```python
from build123d import *

# Parameters (mm, degrees)
FILLET_1_R      = 2
CHAMFER_1_SIZE  = 0.5
CHAMFER_1_SIZE2 = 0.288675135
CHAMFER_2_SIZE  = 0.5
CHAMFER_2_SIZE2 = 0.288675135
SKETCH_2_R      = 17.5
SKETCH_2_R_2    = 10
EXTRUDE_1_DEPTH = 2
CHAMFER_3_SIZE  = 0.5
CHAMFER_4_SIZE  = 0.5
FILLET_2_R      = 0.25


with BuildPart() as part:
    # ｽｹｯﾁ1 → 回転1 (revolve)
    with BuildSketch(Plane(origin=(0, 0, 0), x_dir=(0, 0, -1), z_dir=(1, 0, 0)), mode=Mode.PRIVATE) as revolve_1_sk:
        Polygon((-9, 37.5), (-14, 32.5), (-14, 29), (-7, 29), (-7, 26), (-2, 26), (-2, 12), (3, 12), (3, 17.5), (0, 17.5), (0, 37.5), align=None)
    revolve(revolve_1_sk.sketch.rotate(Axis((0, 0, 26.899509804), (0, 0, -1)), 90), axis=Axis((0, 0, 26.899509804), (0, 0, -1)))

    # ﾌｨﾚｯﾄ1
    fillet_1_edges = [part.edges().sort_by_distance(p)[0] for p in [
        (-17.5, 0, 0),
        (-32.5, 0, 14),
    ]]
    fillet(fillet_1_edges, radius=FILLET_1_R)

    # 面取り1
    chamfer_1_edges = [part.edges().sort_by_distance(p)[0] for p in [
        (-29, 0, 14),
    ]]
    chamfer_1_side = [part.faces().sort_by_distance(p)[0] for p in [
        (-30.775765517, 0, 14),
    ]]
    chamfer(chamfer_1_edges, length=CHAMFER_1_SIZE, length2=CHAMFER_1_SIZE2, reference=chamfer_1_side[0])

    # 面取り2
    chamfer_2_edges = [part.edges().sort_by_distance(p)[0] for p in [
        (-12, 0, 2),
    ]]
    chamfer_2_side = [part.faces().sort_by_distance(p)[0] for p in [
        (-25.264608948, 0, 2),
    ]]
    chamfer(chamfer_2_edges, length=CHAMFER_2_SIZE, length2=CHAMFER_2_SIZE2, reference=chamfer_2_side[0])

    # ｽｹｯﾁ2 → ﾎﾞｽ - 押し出し1 (add)
    with BuildSketch(Plane(origin=(0, 0, -3), x_dir=(-1, 0, 0), z_dir=(0, 0, -1))):
        with Locations(Location((0, 0, 0), (0, 0, 180))):
            Circle(SKETCH_2_R)
        Circle(SKETCH_2_R_2, mode=Mode.SUBTRACT)
    extrude(amount=EXTRUDE_1_DEPTH)

    # 面取り3
    chamfer_3_edges = [part.edges().sort_by_distance(p)[0] for p in [
        (10, 0, -3),
        (10, 0, -5),
    ]]
    chamfer(chamfer_3_edges, length=CHAMFER_3_SIZE)

    # 面取り4
    chamfer_4_edges = [part.edges().sort_by_distance(p)[0] for p in [
        (-37.5, 0, 0),
        (-17.5, 0, -5),
    ]]
    chamfer(chamfer_4_edges, length=CHAMFER_4_SIZE)

    # ﾌｨﾚｯﾄ2
    fillet_2_edges = [part.edges().sort_by_distance(p)[0] for p in [
        (-12, 0, -3),
        (-29, 0, 7),
    ]]
    fillet(fillet_2_edges, radius=FILLET_2_R)


solid = part.part
```
CAD build for the part. Positions are in the model's coordinates, mm. A direction names the side the tool comes from. Round coordinates to 2 decimals unless told otherwise and drop trailing zeros. Loops run counter-clockwise (first coordinate to the right, second up) from the corner with the lowest first, then second, coordinate; pieces in that order, holes last. Notation, with made-up numbers: M 75.5,-8.5 L 125.5,-8.5 A23 cw 125.5,26.5 Z; hole C -7.5,12.25 d5. An arc over 180 degrees is marked long. Use a Markdown table: item, result. Add a question column.
(1) Cut at B-B (z = 5.5). Give the cut face in (x, y).
(2) Cut at A-A (z = 11.25). Give the cut face in (x, y), and give its area (3 significant figures).
(3) Which spindle directions (+Z, -Z, +X, -X, +Y, -Y) get a long thin tool onto all of the face, cutting with end or side? Do faces 1 (the face through (17.3, 33.27, 4.81)), 2 (the face through (-3.794, 17.084, -3.232)), 3 (the face through (11.2, -6.1, 2)). Say none if no direction does.
(4) Flat gauge pins, fed straight in: pin 1 (10 mm diameter, centred on y = 13.5, z = 9, fed in from -X); pin 2 (4 mm diameter, centred on x = -27.5, z = 0, fed in from -Y); pin 3 (8 mm diameter, centred on x = -16, z = 1.5, fed in from +Y). Where does each tip first touch, or does it go through?
(5) Pull direction Y, two halves, no side cores. Call faces 4 (the face through (-20.633, 15.821, 4.465)), 5 (the face through (-16, 16, 0)), 6 (the face through (-7.22, 32.51, 13.2)): +Y half, -Y half, draft (parallel to the pull), parting line (faces both ways), or undercut.
(6) Drill centre lines: line 1 (Y direction, x = 0, z = 5.3); line 2 (Y direction, x = 0, z = -3.9); line 3 (Z direction, x = -23, y = 13.5). Where is each one in solid material? Low to high.
Geometry says:
| question | item | result |
|---|---|---|
| 1 | outline | C 0,0 d75; hole C 0,0 d52 |
| 2 | outline | C 0,0 d70.5; hole C 0,0 d58 |
| 2 | area | 1,260 mm² |
| 3 | face 1 | +Z, -Z |
| 3 | face 2 | -Z |
| 3 | face 3 | +Z |
| 4 | pin 1 | stops at x = -36.52 |
| 4 | pin 2 | stops at y = -27.44 |
| 4 | pin 3 | stops at y = 35.53 |
| 5 | face 4 | undercut |
| 5 | face 5 | draft |
| 5 | face 6 | parting line |
| 6 | line 1 | y = -37.5 to -26, 26 to 37.5 |
| 6 | line 2 | y = -17.5 to -10, 10 to 17.5 |
| 6 | line 3 | z = 0 to 7 |
